from build123d import *

# Parameters (mm, degrees)
F1_DEPTH = 8
F2_R     = 1.6
F3_DEPTH = 25.4


with BuildPart() as f1:
    # F0 (on Top) → F1 (new body)
    with BuildSketch(Plane.XY):
        with BuildLine():
            ThreePointArc((0.5, 6.330284), (0, -6.35), (-0.5, 6.330284))
            Line((-0.5, 6.330284), (-0.5, 13.340633))
            ThreePointArc((-0.5, 13.340633), (-3.057104, 12.995254), (-5.5, 12.164395))
            Line((-5.5, 12.164395), (-5.5, 8.164395))
            Line((-5.5, 8.164395), (-10.562441, 8.164395))
            ThreePointArc((-10.562441, 8.164395), (0, -13.35), (10.562441, 8.164395))
            Line((10.562441, 8.164395), (5.5, 8.164395))
            Line((5.5, 8.164395), (5.5, 12.164395))
            ThreePointArc((5.5, 12.164395), (3.057104, 12.995254), (0.5, 13.340633))
            Line((0.5, 13.340633), (0.5, 6.330284))
        make_face()
    extrude(amount=F1_DEPTH)

    # F2 (on face) → F3 (cut)
    with BuildSketch(Plane.YZ.offset(5.5)):
        with Locations((10.164395, 4)):
            Circle(F2_R)
    extrude(amount=-F3_DEPTH, mode=Mode.SUBTRACT)


solid = f1.part
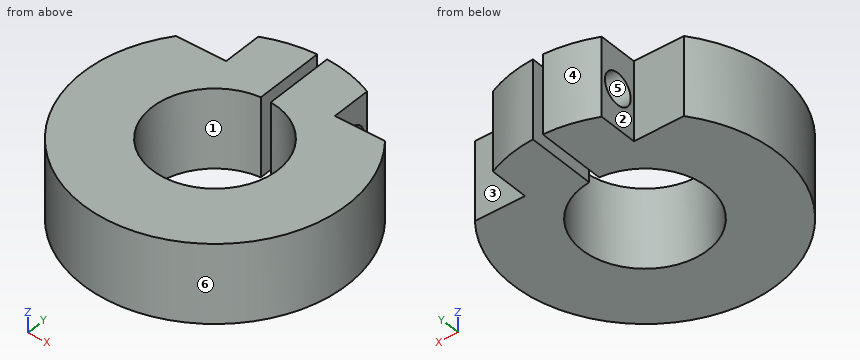
Could you check a few things on this model? Use its own coordinates, in mm. Face numbers are marked on the shaded views. A direction names the side the tool comes from. Coordinates: 2 decimals unless noted, no trailing zeros. Order: outer loops, then holes, each group sorted by start corner. A loop starts at its lowest first (then second) coordinate and runs counter-clockwise, first axis right, second up. Notation, with made-up numbers: (59.5, 74.25) -> (108.5, 74.25) arc R24 ccw to (108.5, 90.25) -> close; hole circle Ø7 at (-34.5, 85). An arc over 180 degrees is marked (long way). One line per item, written item: value. Start each with the question number.
1) Imagine slicing it at A-A on y = 0. List the corners of the cut face in (x, z) for me.
2) Which directions (+Z, -Z, +X, -X, +Y, -Y) give clear straight access to the entire face, cutting with the end or side of a thin tool? Please do the marked faces 1, 2 and 3.
3) Imagine slicing it at D-D on y = 9. List the corners of the cut face in (x, z) for me.
4) Imagine slicing it at C-C on x = -1. List the corners of the cut face in (y, z) for me.
5) We'd pull the mould along Y, two halves only. Please class the marked faces 4, 5 and 6: +Y half, -Y half, draft (parallel to the pull), parting line (faces both ways), or undercut.
6) If I drill on L1, parallel to Y at x = 1, z = 3.25; L2, parallel to X at y = 0, z = 5.5; L3, parallel to X at y = 8.25, z = 7.5, over which ranges is the centre line in solid material (lowest first)? Write a range as [from, to].
7) Imagine slicing it at B-B on z = 7.5. List the corners of the cut face in (x, y) for me.
8) I'm going to push flat-ended pins straight in: pin 1 (3.5 mm diameter, centred on y = 9.5, z = 2.5, fed in from +X); pin 2 (1.5 mm diameter, centred on y = 2, z = 3.5, fed in from -X); pin 3 (4 mm diameter, centred on x = -6, z = 4, fed in from -Y). Where does each tip first touch, or does it pass through?
Answer list:
1. outline: (-13.35, 0) -> (-6.35, 0) -> (-6.35, 8) -> (-13.35, 8) -> close; (6.35, 0) -> (13.35, 0) -> (13.35, 8) -> (6.35, 8) -> close
2. face 1: +Z, -Z
2. face 2: +Z, -Z, -X, +Y
2. face 3: +Z, -Z, +X, +Y
3. outline: (-5.5, 0) -> (-0.5, 0) -> (-0.5, 2.9) -> (-5.5, 2.9) -> close; (-5.5, 5.1) -> (-0.5, 5.1) -> (-0.5, 8) -> (-5.5, 8) -> close; (0.5, 0) -> (5.5, 0) -> (5.5, 2.9) -> (0.5, 2.9) -> close; (0.5, 5.1) -> (5.5, 5.1) -> (5.5, 8) -> (0.5, 8) -> close
4. outline: (-13.31, 0) -> (-6.27, 0) -> (-6.27, 8) -> (-13.31, 8) -> close; (6.27, 0) -> (13.31, 0) -> (13.31, 8) -> (6.27, 8) -> close; hole circle Ø3.2 at (10.16, 4)
5. face 4: +Y half
5. face 5: undercut
5. face 6: parting line
6. L1: y = [-13.31, -6.27], [6.27, 8.75], [11.58, 13.31]
6. L2: x = [-13.35, -6.35], [6.35, 13.35]
6. L3: x = [-5.5, -0.5], [0.5, 5.5]
7. outline: (-10.56, 8.16) arc R13.35 ccw (long way) to (10.56, 8.16) -> (5.5, 8.16) -> (5.5, 12.16) arc R13.35 ccw to (0.5, 13.34) -> (0.5, 6.33) arc R6.35 cw (long way) to (-0.5, 6.33) -> (-0.5, 13.34) arc R13.35 ccw to (-5.5, 12.16) -> (-5.5, 8.16) -> close
8. pin 1: stops at x = 10.87
8. pin 2: stops at x = -13.29
8. pin 3: stops at y = -12.74
